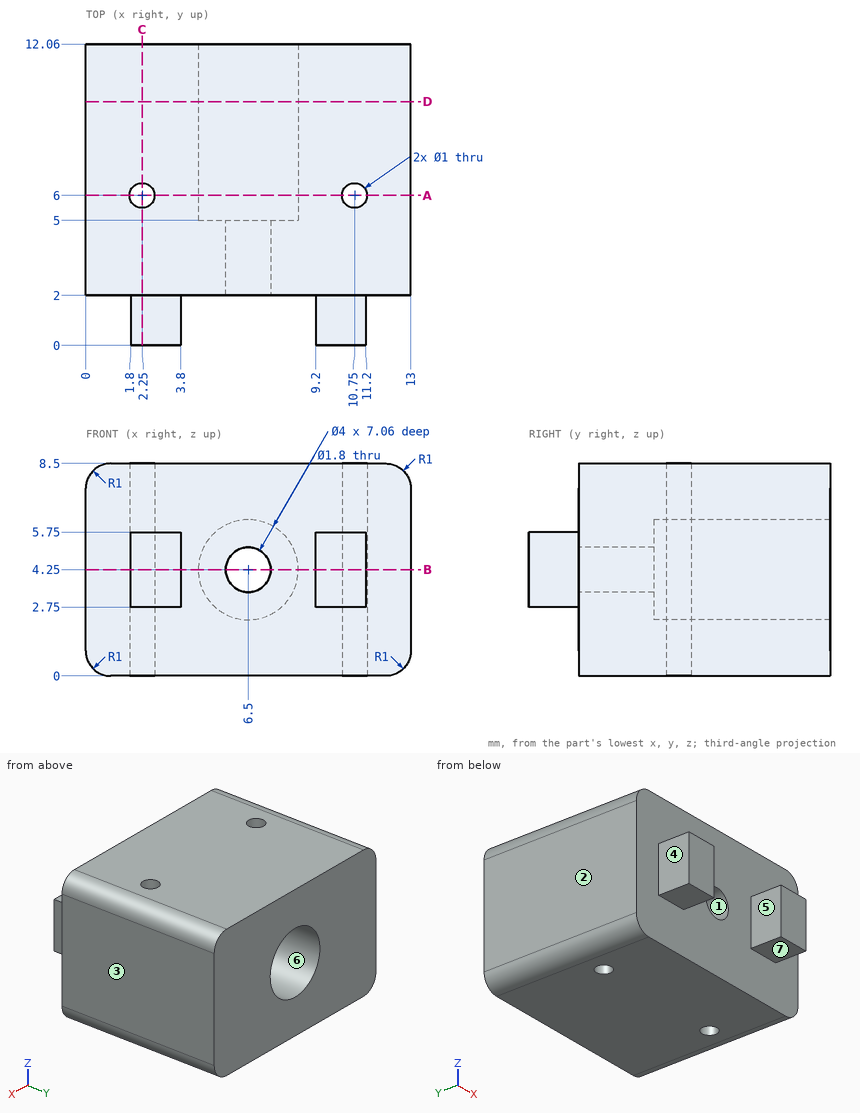
Input: dimensioned drawing with shaded views. Units: mm. Origin: part minimum x, y, z. A direction names the side the tool comes from. Round coordinates to 2 decimals unless told otherwise and drop trailing zeros. Order: outer loops, then holes, each group sorted by start corner. A loop starts at its lowest first (then second) coordinate and runs counter-clockwise, first axis right, second up. Notation, with made-up numbers: (15, -9) -> (19, -9) arc R19 cw to (19, 11) -> close; hole circle Ø10 at (-7.5, 43). An arc over 180 degrees is marked (long way). One line per item, written item: value. Start each with the question number.
Q1. Material intervals for probe 1 along X at (y, z) = (7.5, 4.25); probe 2 along Y at (x, z) = (10.75, 2); probe 3 along Z at (x, y) = (6.5, 7.5), sorted ascending.
Q2. Draft query along X for the marked faces 1, 2 and 3. Return one class per face: pulls with the +X half, pulls with the -X half, needs draft (parallel to the pull), parting line crosses it, or undercut.
Q3. Section query A-A (y = 6). Return the cut outline in (x, z).
Q4. Section query B-B (z = 4.25). Return the cut outline in (x, y), plus the area to 3 significant figures.
Q5. Section query D-D (y = 9.75). Return the cut outline in (x, z).
Q6. Pin query (flat end, axial travel): pin 1 (4 mm diameter, centred on y = 10.5, z = 4, fed in from -X); pin 2 (1.4 mm diameter, centred on x = 6.5, z = 4.25, fed in from -Y); pin 3 (3 mm diameter, centred on x = 7, z = 6.5, fed in from -Y); pin 4 (1.6 mm diameter, centred on y = 1, z = 4.5, fed in from -X). Return the tip coordinate at first contact, or that it passes through.
Q7. Access query for the marked faces 4, 5, 6 and 7. Directions: +Z, -Z, +X, -X, +Y, -Y. A direction counts if a zero-diameter tool reaches every point of the face in a straight line with its end or side. Return the directions, or none.
Q8. Section query C-C (x = 2.25). Return the cut outline in (y, z), plus the area to 3 significant figures.
Findings below:
1. probe 1: 0 to 4.5, 8.5 to 13
1. probe 2: 2 to 5.5, 6.5 to 12.06
1. probe 3: 0 to 2.25, 6.25 to 8.5
2. face 1: undercut
2. face 2: pulls with the -X half
2. face 3: pulls with the +X half
3. outline: (0, 1) arc R1 ccw to (1, 0) -> (1.75, 0) -> (1.75, 8.5) -> (1, 8.5) arc R1 ccw to (0, 7.5) -> close; (2.75, 0) -> (10.25, 0) -> (10.25, 8.5) -> (2.75, 8.5) -> close; (11.25, 0) -> (12, 0) arc R1 ccw to (13, 1) -> (13, 7.5) arc R1 ccw to (12, 8.5) -> (11.25, 8.5) -> close; hole circle Ø4 at (6.5, 4.25)
4. outline: (0, 2) -> (1.8, 2) -> (1.8, 0) -> (3.8, 0) -> (3.8, 2) -> (5.6, 2) -> (5.6, 5) -> (4.5, 5) -> (4.5, 12.06) -> (0, 12.06) -> close; (7.4, 2) -> (9.2, 2) -> (9.2, 0) -> (11.2, 0) -> (11.2, 2) -> (13, 2) -> (13, 12.06) -> (8.5, 12.06) -> (8.5, 5) -> (7.4, 5) -> close; hole circle Ø1 at (2.25, 6); hole circle Ø1 at (10.75, 6)
4. area: 104 mm²
5. outline: (0, 1) arc R1 ccw to (1, 0) -> (12, 0) arc R1 ccw to (13, 1) -> (13, 7.5) arc R1 ccw to (12, 8.5) -> (1, 8.5) arc R1 ccw to (0, 7.5) -> close; hole circle Ø4 at (6.5, 4.25)
6. pin 1: x = 0
6. pin 2: through
6. pin 3: y = 2
6. pin 4: x = 1.8
7. face 4: +Z, -Z, -X, -Y
7. face 5: +Z, -Z, -Y
7. face 6: +Y
7. face 7: -Z, +X, -X, -Y
8. outline: (0, 2.75) -> (2, 2.75) -> (2, 0) -> (5.5, 0) -> (5.5, 8.5) -> (2, 8.5) -> (2, 5.75) -> (0, 5.75) -> close; (6.5, 0) -> (12.06, 0) -> (12.06, 8.5) -> (6.5, 8.5) -> close
8. area: 83.0 mm²
